Check sheet for the modelled part. Datum: model origin and axes. Units: mm. Face numbers are marked on the shaded views. A direction names the side the tool comes from. Coordinates: 2 decimals unless noted, no trailing zeros. Loops run counter-clockwise (first coordinate to the right, second up) from the corner with the lowest first, then second, coordinate; pieces in that order, holes last.
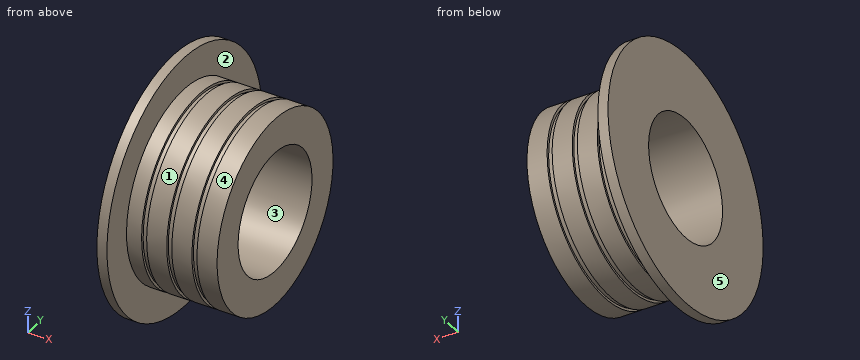
```python
from build123d import *

# Parameters (mm, degrees)
SKETCH2_W = 1
SKETCH2_H = 0.5


with BuildPart() as part:
    # Sketch1 → Revolve1 (revolve)
    with BuildSketch(Plane.XY, mode=Mode.PRIVATE) as revolve1_sk:
        Polygon((10.740740741, -3.925925926), (-9.259259259, -3.925925926), (-9.259259259, 9.249074074), (-7.259259259, 9.249074074), (-7.259259259, 2.899074074), (10.740740741, 2.899074074), align=None)
    revolve(revolve1_sk.sketch.rotate(Axis((-9.259259259, -15.925925926, 0), (1, 0, 0)), 90), axis=Axis((-9.259259259, -15.925925926, 0), (1, 0, 0)))

    # Sketch2 → Cut-Revolve1 (revolve, cut)
    with BuildSketch(Plane.XY, mode=Mode.PRIVATE) as cut_revolve1_sk:
        with Locations((6.240740741, 2.649074074)):
            Rectangle(SKETCH2_W, SKETCH2_H)
        with Locations((1.240740741, 2.649074074)):
            Rectangle(SKETCH2_W, SKETCH2_H)
        with Locations((-3.759259259, 2.649074074)):
            Rectangle(SKETCH2_W, SKETCH2_H)
    revolve(cut_revolve1_sk.sketch.rotate(Axis((10.740740741, -15.925925926, 0), (-1, 0, 0)), 90), axis=Axis((10.740740741, -15.925925926, 0), (-1, 0, 0)), mode=Mode.SUBTRACT)


solid = part.part
```
1) Section check B-B on x = 4.75. Enter the section's corners in (y, z) (3 decimals), plus the area to 3 significant figures.
Answer sheet:
outline: circle Ø37.65 at (-15.926, 0); hole circle Ø24 at (-15.926, 0)
area: 661 mm2
2) Depth check by flat-ended pin: pin 1 (10 mm diameter, centred on x = 1, y = -20.5, fed in from -Z) (3 decimals); pin 2 (12 mm diameter, centred on x = 8.5, y = 0.5, fed in from -Z); pin 3 (6 mm diameter, centred on x = -5, y = -9, fed in from +Z); pin 4 (6 mm diameter, centred on y = -21.5, z = 4.5, fed in from -X). Enter the tip coordinate at first touch or a pass-through.
Answer sheet:
pin 1: stops at z = -18.825
pin 2: stops at z = -15.67
pin 3: stops at z = 24.68
pin 4: passes through
3) Set-up check for the marked faces 4 and 5: record each of +Z, -Z, +X, -X, +Y, -Y from which the full face is reachable in a straight line by a thin tool's end or side.
Answer sheet:
face 4: +X
face 5: +Z, -Z, -X, +Y, -Y
4) Scan lines: line 1 (Y direction, x = 6, z = 0); line 2 (Z direction, x = 5, y = -16.5); line 3 (Y direction, x = -1.75, z = 0). Record each from-to range of solid material in increasing order.
Answer sheet:
line 1: y = -34.25 to -27.93, -3.93 to 2.4
line 2: z = -18.82 to -11.99, 11.99 to 18.82
line 3: y = -34.75 to -27.93, -3.93 to 2.9
5) Section check C-C on y = 3.5. Enter the section's corners in (x, z).
Answer sheet:
outline: (-9.26, -16.01) - (-7.26, -16.01) - (-7.26, 16.01) - (-9.26, 16.01) - close
6) Mould release check, pull along Y, two halves, no side actions. Record for the marked faces 1, 2 and 3: +Y half, -Y half, draft (parallel to the pull), parting line (faces both ways), or undercut.
Answer sheet:
face 1: parting line
face 2: draft
face 3: undercut
